The drawing under review shows one solid part. Ordinate dimensions are in mm from its lowest x, y, z. Round coordinates to 2 decimals unless told otherwise and drop trailing zeros. Write each loop counter-clockwise with the first axis right and the second up, starting at its lowest first coordinate (ties: lowest second). Pieces come first, ordered by that corner, then holes. Notation, with made-up numbers: M 14.5,48.5 L 26.5,48.5 A12 ccw 26.5,57.5 Z; hole C -35.5,65.5 d3. An arc over 180 degrees is marked long. One line per item, written item: value. Start each with the question number.
1) Mouldability with a two-part tool opening along Z and no side actions: class the marked faces 1, 2, 3 and 4 as +Z half, -Z half, draft (parallel to the pull), parting line (faces both ways), or undercut.
2) For P1, Ø2, axis at x = 7, y = 1.5, coming from the -Z side, flat-tipped, find the tip position at first contact; note if it passes through.
3) Take a section at A-A, the plane y = 3.5. Write out the cut boundary in (x, z) (1 decimal), and give its area (3 significant figures).
4) Wall thickness on probe 1 along X at (y, z) = (6.75, 8.5); probe 2 along Z at (x, y) = (4.5, 2) (1 decimal); probe 3 along Z at (x, y) = (5, 5) (1 decimal): over which ranges is each line inside the solid? List them lowest first.
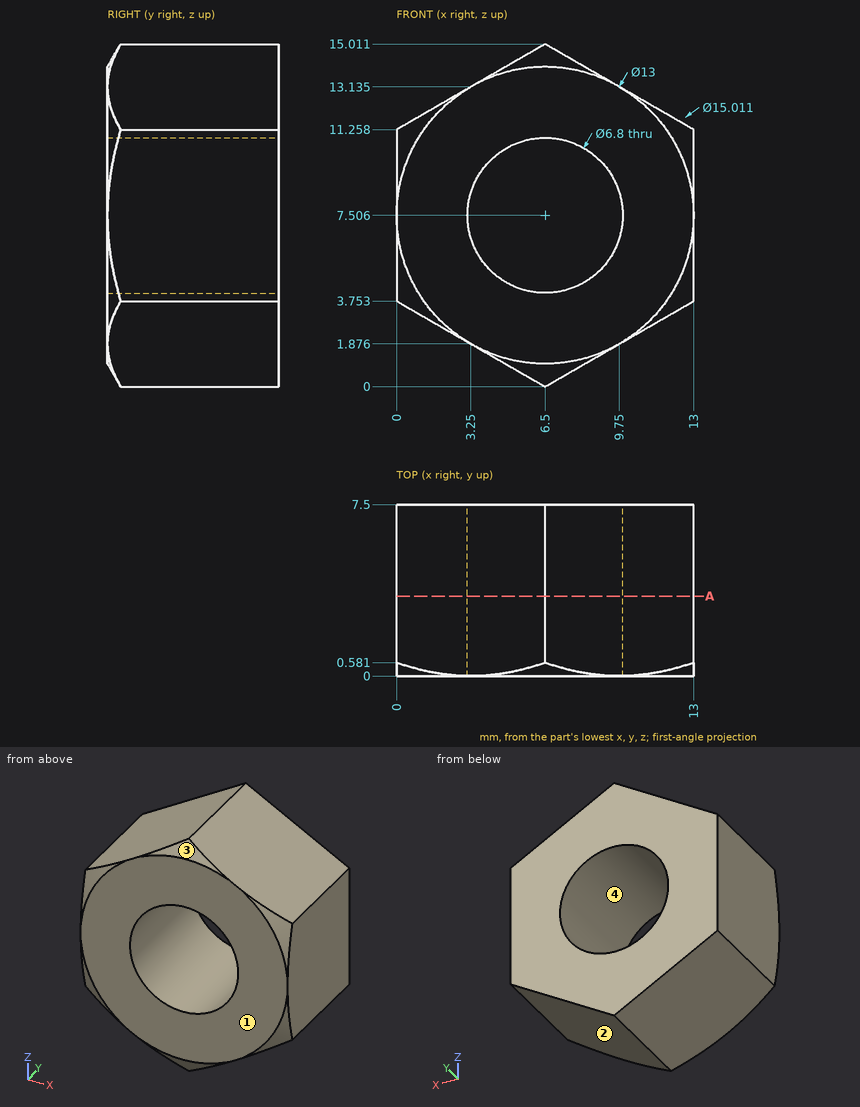
Checked values:
1. face 1: draft
1. face 2: -Z half
1. face 3: +Z half
1. face 4: undercut
2. P1: stops at z = 0
3. outline: M 0,3.8 L 6.5,0 L 13,3.8 L 13,11.3 L 6.5,15 L 0,11.3 Z; hole C 6.5,7.5 d6.8
3. area: 110 mm2
4. probe 1: x = 0 to 3.25, 9.75 to 13
4. probe 2: z = 1.2 to 4.8, 10.3 to 13.9
4. probe 3: z = 0.9 to 4.5, 10.6 to 14.1
